Here's how the part is built. I have some questions about the finished solid (model axes, mm). A direction names the side the tool comes from. Round coordinates to 2 decimals unless told otherwise and drop trailing zeros. Order: outer loops, then holes, each group sorted by start corner. A loop starts at its lowest first (then second) coordinate and runs counter-clockwise, first axis right, second up. Notation, with made-up numbers: M -19,39 L -15,39 A13 ccw -15,58 Z; hole C 0.25,-31.5 d7. An arc over 180 degrees is marked long. Write item = value, one per line. Start each with the question number.
Item 1: I want a section at B-B, the plane y = 24. List the corners of the cut face in (x, z) for me, plus the area to 3 significant figures.
Item 2: Please list where these lines run through material, in increasing order: L1, parallel to X at y = 2, z = 3.5; L2, parallel to Z at x = 23, y = 6; L3, parallel to Z at x = 7, y = 3.5.
Item 3: I want a section at A-A, the plane y = 6. List the corners of the cut face in (x, z) for me.
Item 4: I want a section at C-C, the plane z = 9.25. List the corners of the cut face in (x, y) for me.
Item 5: For faces 4 (the face through (9, 32, 0)), 5 (the face through (5, 22, 0)), 6 (the face through (12, 20, 10)), which set-ups out of +Z, -Z, +X, -X, +Y, -Y let a thin tool reach every point of the face, with its end or its side?
Item 6: We'd pull the mould along X, two halves only. Please class faces 1 (the face through (22.486, 6.26, 11.233)), 2 (the face through (7.93, 31.86, 13.23)), 3 (the face through (-7.5, 22, 1.2)): pulls with the +X half, pulls with the -X half, needs draft (parallel to the pull), parting line crosses it, or undercut.
Item 7: I'm going to push flat-ended pins straight in: P1, Ø1.5, axis at x = 9, z = 6, coming from the -Y side; P2, Ø5, axis at y = 32.5, z = 2.5, coming from the +X side; P3, Ø3, axis at x = -3, y = 28.5, coming from the +Z side; P4, Ø6, axis at x = 0.5, z = 12.5, coming from the -Y side. Where does each tip first touch, or does it pass through?
Item 8: I want a section at D-D, the plane x = 10.5. List the corners of the cut face in (y, z) for me, plus the area to 3 significant figures.
```python
from build123d import *

# Parameters (mm, degrees)
F1_DEPTH     = 20
F2_R         = 2
F3_R         = 4
F5_DEPTH     = 1.5
F6_R         = 8
F7_DEPTH     = 20
F8_DEPTH     = 25
F9_W         = 5
F9_H         = 35.9879870677
F9_H_2       = 3.0384219572
F9_H_3       = 2
F10_DEPTH    = 12.4
F11_T1_DEPTH = 26.8776444438
F12_R        = 1
F13_R        = 5
F15_DEPTH    = 20
F17_DEPTH    = 20
F18_R        = 30
F19_R        = 2
F20_DEPTH    = 58


# Not quite as in the source:
# - a fillet or chamfer that OpenCascade refuses, or shapes differently, is made with other operations: its cross-section is extruded or revolved along the edge and cut away or added
# - ends of sketch curves that miss each other by under 0.0002 mm in the source are joined


with BuildPart() as f1:
    # F0 (on Top) → F1 (new body)
    with BuildSketch(Plane.XY):
        Polygon((-21.4999990134, 20), (21.5000009866, 20), (21.5, 0), (23.5, 0), (23.5000010853, 22), (-23.4999989147, 22), (-23.5, 0), (-21.5, 0), align=None)
    extrude(amount=F1_DEPTH)

    # F2
    f2_edges = [f1.edges().sort_by_distance(p)[0] for p in [
        (-21.499999, 20, 10),
        (21.500001, 20, 10),
    ]]
    fillet(f2_edges, radius=F2_R)

    # F3
    f3_edges = [f1.edges().sort_by_distance(p)[0] for p in [
        (-23.499999, 22, 10),
        (23.500001, 22, 10),
    ]]
    fillet(f3_edges, radius=F3_R)

    # F4 (on face) → F5 (join)
    with BuildSketch(Plane(origin=(0, 0, 0), x_dir=(1, 0, 0), z_dir=(0, 0, -1))):
        with BuildLine():
            Line((21.500000888, -17.9999999013), (21.5, 0))
            Line((21.5, 0), (-21.5, -2.2199e-06))
            Line((-21.5, -2.2199e-06), (-21.499999112, -18.0000000987))
            ThreePointArc((-21.499999112, -18.0000000987), (-20.9142126395, -19.4142135973), (-19.499999112, -20))
            Line((-19.499999112, -20), (19.500000888, -20))
            ThreePointArc((19.500000888, -20), (20.9142144852, -19.4142135275), (21.500000888, -17.9999999013))
        make_face()
        with BuildLine():
            ThreePointArc((19.500000888, -22), (22.3284280825, -20.828427055), (23.500000888, -17.9999998027))
            Line((23.500000888, -17.9999998027), (23.5, 0))
            Line((23.5, 0), (21.5, -9.87e-08))
            Line((21.5, -9.87e-08), (21.500000888, -17.9999999013))
            ThreePointArc((21.500000888, -17.9999999013), (20.9142144852, -19.4142135275), (19.500000888, -20))
            Line((19.500000888, -20), (-19.499999112, -20))
            ThreePointArc((-19.499999112, -20), (-20.9142126395, -19.4142135973), (-21.499999112, -18.0000000987))
            Line((-21.499999112, -18.0000000987), (-21.5, 0))
            Line((-21.5, 0), (-23.5, -2.3186e-06))
            Line((-23.5, -2.3186e-06), (-23.499999112, -18.0000001973))
            ThreePointArc((-23.499999112, -18.0000001973), (-22.328426167, -20.8284271945), (-19.499999112, -22))
            Line((-19.499999112, -22), (19.500000888, -22))
        make_face()
    extrude(amount=F5_DEPTH)

    # F6 (on face) → F7 (join)
    with BuildSketch(Plane(origin=(0, 22, 0), x_dir=(-1, 0, 0), z_dir=(0, 1, 0))):
        with BuildLine():
            ThreePointArc((4.21e-08, -1.5), (6.7175144362, 1.2824855936), (9.5, 8))
            ThreePointArc((9.5, 8), (-6.7175144362, 14.7175144064), (4.21e-08, -1.5))
        make_face()
        with Locations((0, 8)):
            Circle(F6_R, mode=Mode.SUBTRACT)
    extrude(amount=F7_DEPTH)

    # F8 (cut): a face of the model
    f8_faces = [f1.faces().sort_by_distance(p)[0] for p in [
        (0, 22, 8),
    ]]
    extrude(f8_faces, amount=-F8_DEPTH, mode=Mode.SUBTRACT)

    # F9 (on face) → F10 (cut)
    with BuildSketch(Plane.XY.offset(20)):
        with Locations((0, 39.9939935338)):
            Rectangle(F9_W, F9_H)
        with Locations((0, 18.4807890214)):
            Rectangle(F9_W, F9_H_2)
        with Locations((0, 21)):
            Rectangle(F9_W, F9_H_3)
    extrude(amount=-F10_DEPTH, mode=Mode.SUBTRACT)

    # F11: chamfer of 1 on 2 edges, made by hand

    # F11_s2 → F11_t1 (cut)
    with BuildSketch(Plane.XZ.offset(-44.4388222219)):
        with BuildLine():
            Line((-3.3316740869, 15.2494859065), (-2.4783436331, 16.5746305544))
            Line((-2.4783436331, 16.5746305544), (-2.4583436331, 16.5746305544))
            ThreePointArc((-2.4583436331, 16.5746305544), (-2.48, 16.0869863156), (-2.48, 15.5993420768))
            Line((-2.48, 15.5993420768), (-2.49375, 15.5803437216))
            ThreePointArc((-2.49375, 15.5803437216), (-2.9171284808, 15.4277022979), (-3.3233990426, 15.2312781158))
            Line((-3.3233990426, 15.2312781158), (-3.3316740869, 15.2494859065))
        make_face()
        with BuildLine():
            Line((2.4783436331, 16.5746305544), (3.3316740869, 15.2494859065))
            Line((3.3316740869, 15.2494859065), (3.3233990426, 15.2312781158))
            ThreePointArc((3.3233990426, 15.2312781158), (2.9171284808, 15.4277022979), (2.49375, 15.5803437216))
            Line((2.49375, 15.5803437216), (2.48, 15.5993420768))
            ThreePointArc((2.48, 15.5993420768), (2.48, 16.0869863156), (2.4583436331, 16.5746305544))
            Line((2.4583436331, 16.5746305544), (2.4783436331, 16.5746305544))
        make_face()
    extrude(amount=F11_T1_DEPTH, mode=Mode.SUBTRACT)

    # F12
    f12_edges = [f1.edges().sort_by_distance(p)[0] for p in [
        (2.5, 21, 20),
        (-2.5, 21, 20),
    ]]
    fillet(f12_edges, radius=F12_R)

    # F13
    f13_edges = [f1.edges().sort_by_distance(p)[0] for p in [
        (-22.5, 0, 20),
        (22.5, 0, 20),
    ]]
    fillet(f13_edges, radius=F13_R)

    # F14 (on face) → F15 (join)
    with BuildSketch(Plane(origin=(0, 22, 0), x_dir=(-1, 0, 0), z_dir=(0, 1, 0))):
        with BuildLine():
            ThreePointArc((2.1e-08, -1.5), (-5.5388120473, 0.2817384662), (-9, 4.9586187349))
            Line((-9, 4.9586187349), (-9, -1.5))
            Line((-9, -1.5), (0, -1.5))
        make_face()
        with BuildLine():
            ThreePointArc((9, 4.9586187349), (5.5388120644, 0.2817384785), (2.1e-08, -1.5))
            Line((0, -1.5), (9, -1.5))
            Line((9, -1.5), (9, 4.9586187349))
        make_face()
    extrude(amount=F15_DEPTH)

    # F16 (on face) → F17 (cut)
    with BuildSketch(Plane(origin=(0, 42, 0), x_dir=(-1, 0, 0), z_dir=(0, 1, 0))):
        with BuildLine():
            ThreePointArc((-7, 2.3431457505), (-7.53910447, 3.0845240526), (-8, 3.8768943744))
            Line((-8, 3.8768943744), (-8, -0.5))
            Line((-8, -0.5), (-7, -0.5))
            Line((-7, -0.5), (-7, 2.3431457505))
        make_face()
        with BuildLine():
            Line((8, -0.5), (8, 3.8768943744))
            ThreePointArc((8, 3.8768943744), (7.53910447, 3.0845240526), (7, 2.3431457505))
            Line((7, 2.3431457505), (7, -0.5))
            Line((7, -0.5), (8, -0.5))
        make_face()
        with BuildLine():
            ThreePointArc((-4.8538187839, 0.4210526316), (-5.4443451471, 0.8334732318), (-6, 1.2917960675))
            Line((-6, 1.2917960675), (-6, -0.5))
            Line((-6, -0.5), (-5.123475383, -0.5))
            ThreePointArc((-5.123475383, -0.5), (-4.643617948, -0.1404878717), (-4.8538187839, 0.4210526316))
        make_face()
        with BuildLine():
            Line((6, -0.5), (6, 1.2917960675))
            ThreePointArc((6, 1.2917960675), (5.4443451471, 0.8334732318), (4.8538187839, 0.4210526316))
            ThreePointArc((4.8538187839, 0.4210526316), (4.643617948, -0.1404878717), (5.123475383, -0.5))
            Line((5.123475383, -0.5), (6, -0.5))
        make_face()
    extrude(amount=-F17_DEPTH, mode=Mode.SUBTRACT)

    # F18
    f18_edges = [f1.edges().sort_by_distance(p)[0] for p in [
        (-9, 32, 4.958619),
        (9, 32, 4.958619),
    ]]
    fillet(f18_edges, radius=F18_R)

    # F19 (on face) → F20 (cut)
    with BuildSketch(Plane(origin=(-23.5, 1.1593e-06, 0), x_dir=(-4.93e-08, -1, 0), z_dir=(-1, 4.93e-08, 0))):
        with Locations((-5.999999038, 9.25)):
            Circle(F19_R)
    extrude(amount=-F20_DEPTH, mode=Mode.SUBTRACT)


solid = f1.part
```
Filled in:
q1.outline = M -9.38,6.49 A30 cw -9,1.74 L -9,-1.5 L 9,-1.5 L 9,1.74 A30 cw 9.38,6.49 A9.5 ccw 2.5,17.17 L 2.5,16.54 L 3.31,15.28 A8 cw long -3.31,15.28 L -2.5,16.54 L -2.5,17.17 A9.5 ccw Z; hole M -8,-0.5 L -7,-0.5 L -7,2.34 A9 cw -8,3.88 Z; hole M -6,-0.5 L -5.12,-0.5 A0.5 ccw -4.85,0.42 A9 cw -6,1.29 Z; hole M 4.85,0.42 A0.5 ccw 5.12,-0.5 L 6,-0.5 L 6,1.29 A9 cw Z; hole M 7,-0.5 L 8,-0.5 L 8,3.88 A9 cw 7,2.34 Z
q1.area = 95.5 mm^2
q2.L1 = -23.5 to -21.5, 21.5 to 23.5
q2.L2 = -1.5 to 7.25, 11.25 to 20
q2.L3 = -1.5 to 0
q3.outline = M -23.5,-1.5 L 23.5,-1.5 L 23.5,7.25 L 21.5,7.25 L 21.5,0 L -21.5,0 L -21.5,7.25 L -23.5,7.25 Z; M -23.5,11.25 L -21.5,11.25 L -21.5,20 L -23.5,20 Z; M 21.5,11.25 L 23.5,11.25 L 23.5,20 L 21.5,20 Z
q4.outline = M -23.5,0 L -21.5,0 L -21.5,4 L -23.5,4 Z; M -23.5,8 L -21.5,8 L -21.5,18 A2 cw -19.5,20 L -7.9,20 L -7.9,42 L -9.42,42 L -9.42,22 L -19.5,22 A4 ccw -23.5,18 Z; M 7.9,20 L 19.5,20 A2 cw 21.5,18 L 21.5,8 L 23.5,8 L 23.5,18 A4 ccw 19.5,22 L 9.42,22 L 9.42,42 L 7.9,42 Z; M 21.5,0 L 23.5,0 L 23.5,4 L 21.5,4 Z
q5.face_4 = -Z, +X, +Y
q5.face_5 = +Y
q5.face_6 = +Z, -Y
q6.face_1 = needs draft
q6.face_2 = pulls with the +X half
q6.face_3 = undercut
q7.P1 = 20
q7.P2 = 9.18
q7.P3 = 17.17
q7.P4 = through
q8.outline = M 0,-1.5 L 22,-1.5 L 22,20 L 20,20 L 20,0 L 0,0 Z
q8.area = 73.0 mm^2
